Check sheet for the modelled part. Datum: model origin and axes. Units: mm. Give positions to 0.01 mm unless a question says otherwise; leave off trailing zeros. Order: outer loops, then holes, each group sorted by start corner. A loop starts at its lowest first (then second) coordinate and runs counter-clockwise, first axis right, second up. Notation, with made-up numbers: (21.25, -29.75) -> (76.25, -29.75) arc R26 ccw to (76.25, -14.75) -> close; hole circle Ø5 at (39.5, 63). An arc over 180 degrees is marked (long way). Answer in a Markdown table with one row per item. Add a question column.
(1) Cross-section at B-B (x = 2). State how many separate pieces and enclosed holes the cut face has, then the cut area to 3 significant figures.
(2) Cross-section at A-A (z = 5.5). Record the cut outline in (x, y).
(3) Go/stop test with flat-tipped pins: pin 1 (2 mm diameter, centred on x = -11.5, y = 30, fed in from -Z); pin 2 (1.5 mm diameter, centred on x = 30, y = -6, fed in from +Z) (3 decimals); pin 3 (21 mm diameter, centred on x = -9, y = -1.5, fed in from +Z); pin 4 (6 mm diameter, centred on y = -8, z = 2, fed in from +X). Record where each tip stops, or that it passes through.
(4) Thickness scan on L1, parallel to Y at x = 0, z = 1.9; L2, parallel to Y at x = 0, z = 1.05; L3, parallel to Z at x = 9, y = 30 (3 decimals). Record the ranges inside material, lowest first. Write a range as [from, to].
```python
from build123d import *

# Parameters (mm, degrees)
F0_R     = 0.762
F0_R_2   = 14.3129
F1_DEPTH = 3.175
F2_R     = 2.54
F3_DEPTH = 12.7


with BuildPart() as f1:
    # F0 (on Top) → F1 (new body)
    with BuildSketch(Plane.XY):
        with BuildLine():
            ThreePointArc((37.814818885, -4.6528993857), (16.2183640692, 8.713670097), (16.9939270688, 34.1000944688))
            ThreePointArc((16.9939270688, 34.1000944688), (1.1909176957, 38.0813827879), (-14.8299813197, 35.0953223957))
            ThreePointArc((-14.8299813197, 35.0953223957), (-15.6508840085, 9.7188762367), (-38.0323831061, -2.2688841474))
            ThreePointArc((-38.0323831061, -2.2688841474), (-33.5888120947, -17.9833729335), (-22.9742885145, -30.3939478721))
            ThreePointArc((-22.9742885145, -30.3939478721), (-0.5866848831, -18.4058352173), (20.9920077442, -31.7953709031))
            ThreePointArc((20.9920077442, -31.7953709031), (32.3842423806, -20.0716428185), (37.814818885, -4.6528993857))
        make_face()
        with BuildLine():
            ThreePointArc((-22.6742041591, -21.077906737), (-30.5143778905, -16.2115761649), (-30.2921493088, -6.9866039788))
            Line((-30.2921493088, -6.9866039788), (-22.6742041591, -21.077906737))
        make_face(mode=Mode.SUBTRACT)
        with Locations((-9.7768361415, -15.7612173143)):
            Circle(F0_R, mode=Mode.SUBTRACT)
        with BuildLine():
            ThreePointArc((-22.077246757, -2.5455187134), (-14.2471455868, -7.4172946457), (-14.4593016073, -16.6368214716))
            Line((-14.4593016073, -16.6368214716), (-22.077246757, -2.5455187134))
        make_face(mode=Mode.SUBTRACT)
        with Locations((8.761196518, -16.3475971243)):
            Circle(F0_R, mode=Mode.SUBTRACT)
        with BuildLine():
            ThreePointArc((12.5619529023, -18.1867123268), (12.756507598, -9.1097250706), (20.6001486004, -4.5373247159))
            Line((20.6001486004, -4.5373247159), (12.5619529023, -18.1867123268))
        make_face(mode=Mode.SUBTRACT)
        with Locations((18.5380326595, -0.58637981)):
            Circle(F0_R, mode=Mode.SUBTRACT)
        with BuildLine():
            Line((20.8666791326, -23.0774090058), (28.9048748307, -9.4280213948))
            ThreePointArc((28.9048748307, -9.4280213948), (28.7016006579, -18.4998737054), (20.8666791326, -23.0774090058))
        make_face(mode=Mode.SUBTRACT)
        with Locations((-18.5380326595, 0.58637981)):
            Circle(F0_R, mode=Mode.SUBTRACT)
        with Locations((-8.761196518, 16.3475971243)):
            Circle(F0_R, mode=Mode.SUBTRACT)
        Circle(F0_R_2, mode=Mode.SUBTRACT)
        with BuildLine():
            ThreePointArc((8.554840384, 20.4151336434), (0.3927024044, 16.1488375122), (-7.4634526605, 20.9553546163))
            Line((-7.4634526605, 20.9553546163), (8.554840384, 20.4151336434))
        make_face(mode=Mode.SUBTRACT)
        with Locations((9.7768361415, 15.7612173143)):
            Circle(F0_R, mode=Mode.SUBTRACT)
        with BuildLine():
            Line((8.86910012, 29.7333659897), (-7.1491929245, 30.2735869625))
            ThreePointArc((-7.1491929245, 30.2735869625), (1.0136418787, 34.5605448721), (8.86910012, 29.7333659897))
        make_face(mode=Mode.SUBTRACT)
    extrude(amount=F1_DEPTH)

    # F2
    f2_edges = [f1.edges().sort_by_distance(p)[0] for p in [
        (-15.650884, 9.718876, 0),
        (1.190918, 38.081383, 0),
        (-0.586685, -18.405835, 0),
        (32.384242, -20.071643, 0),
        (16.218364, 8.71367, 0),
        (-33.588812, -17.983373, 0),
    ]]
    fillet(f2_edges, radius=F2_R)

    # F0 (on Top) → F3 (join)
    with BuildSketch(Plane.XY):
        with Locations((-8.761196518, 16.3475971243)):
            Circle(F0_R)
        with Locations((-18.5380326595, 0.58637981)):
            Circle(F0_R)
        with Locations((-9.7768361415, -15.7612173143)):
            Circle(F0_R)
        with Locations((8.761196518, -16.3475971243)):
            Circle(F0_R)
        with Locations((18.5380326595, -0.58637981)):
            Circle(F0_R)
        with Locations((9.7768361415, 15.7612173143)):
            Circle(F0_R)
    extrude(amount=F3_DEPTH)


solid = f1.part
```
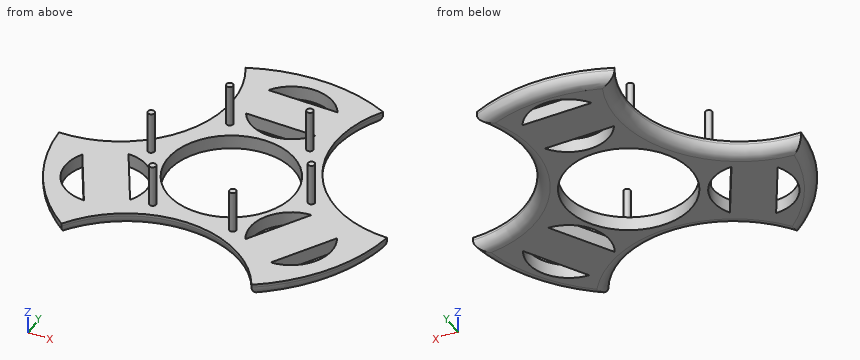
Answer below:
| question | item | result |
|---|---|---|
| 1 | separate pieces | 4 |
| 1 | enclosed holes | 0 |
| 1 | area | 58.8 mm² |
| 2 | outline | circle Ø1.52 at (-18.54, 0.59); circle Ø1.52 at (-9.78, -15.76); circle Ø1.52 at (-8.76, 16.35); circle Ø1.52 at (8.76, -16.35); circle Ø1.52 at (9.78, 15.76); circle Ø1.52 at (18.54, -0.59) |
| 3 | pin 1 | stops at z = 0.02 |
| 3 | pin 2 | stops at z = 3.175 |
| 3 | pin 3 | stops at z = 12.7 |
| 3 | pin 4 | stops at x = 37.76 |
| 4 | L1 | y = [-18.35, -14.31], [14.31, 16.17], [20.7, 30.03], [34.54, 38.02] |
| 4 | L2 | y = [-17.95, -14.31], [14.31, 16.17], [20.7, 30.03], [34.54, 37.62] |
| 4 | L3 | z = [0, 3.175] |
